Input: dimensioned drawing with shaded views. Units: mm. Origin: part minimum x, y, z. A direction names the side the tool comes from. Round coordinates to 2 decimals unless told otherwise and drop trailing zeros. Loops run counter-clockwise (first coordinate to the right, second up) from the corner with the lowest first, then second, coordinate; pieces in that order, holes last. Notation, with made-up numbers: M 34,33.5 L 41,33.5 A12 ccw 41,54.5 Z; hole C 88.25,20.25 d6. An arc over 180 degrees is marked long. Write each question's results on one line, items separated by ' | '. Start each with the question number.
1. Draft query along X for the marked faces 1, 2, 3 and 4. Return one class per face: released by +X, released by -X, zero draft, split by the parting line, or undercut.
2. Section A-A on z = 1. Output: boundary loops of the cut face in (x, y), and give its area (3 significant figures).
3. Section D-D on x = 9.75. Output: boundary loops of the cut face in (y, z), and give its area (3 significant figures).
4. Contact query for flat-ended pins moving along their axis: pin 1 Ø0.5 at (x, y) = (11.5, 8) entering from +Z; pin 2 Ø1.5 at (x, z) = (6.5, 6) entering from +Y; pin 3 Ø1.1 at (y, z) = (9.5, 2) entering from -X; pin 4 Ø3.5 at (x, y) = (5, 5) entering from -Z. Output: stop coordinate, or through.
5. Ray query, line 1 (X direction, y = 4.5, z = 4.75); line 2 (Z direction, x = 2.75, y = 8.5); line 3 (Y direction, x = 10, z = 3.25). Return the intervals inside material, ascending.
6. Section C-C on y = 7.75. Output: boundary loops of the cut face in (x, z).
7. Section B-B on x = 3.5. Output: boundary loops of the cut face in (y, z), and give its area (3 significant figures).
8. Set-up query: the marked faces 5, 6, 7, 8 and 9. Return all of +Z, -Z, +X, -X, +Y, -Y with unobstructed straight access to the full face (end or side cutting, diameter ignored); none if empty.
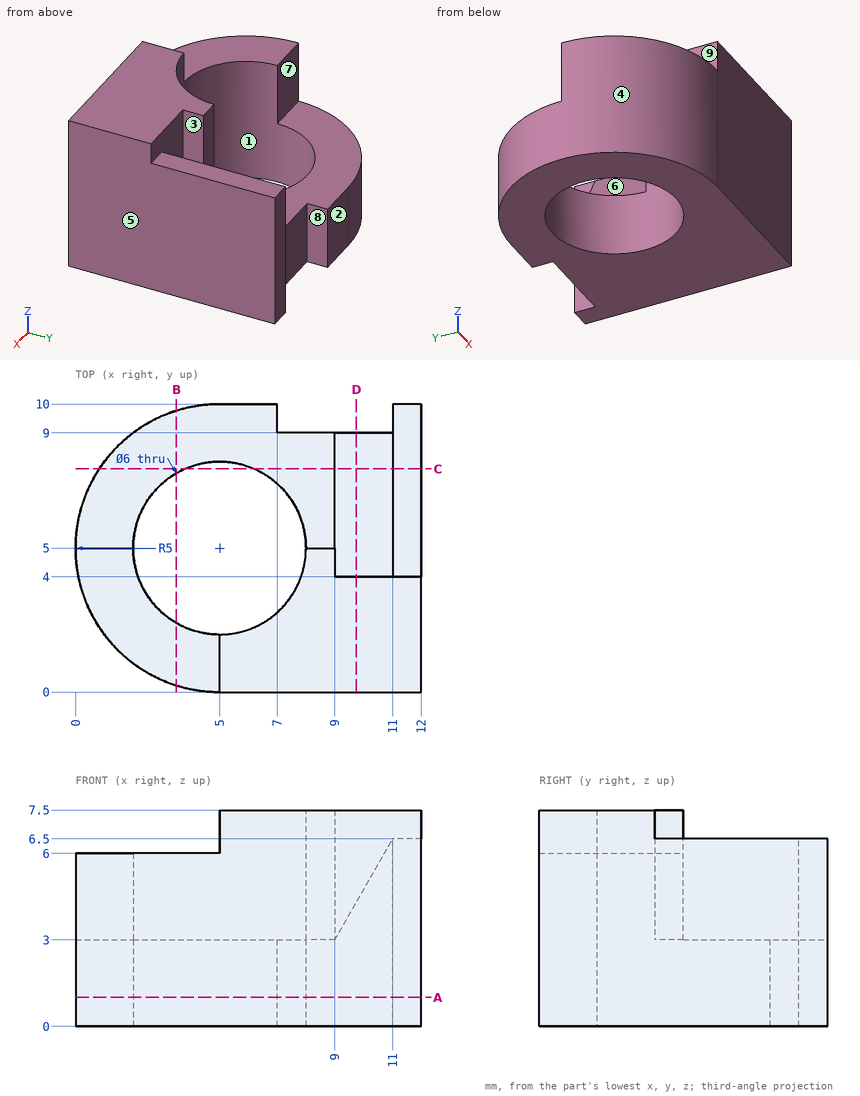
Taken from the geometry:
1) face 1: undercut | face 2: zero draft | face 3: undercut | face 4: released by -X
2) outline: M 5,0 L 12,0 L 12,10 L 11,10 L 11,9 L 7,9 L 7,10 L 5,10 A5 ccw Z; hole C 5,5 d6 | area: 77.0 mm^2
3) outline: M 0,0 L 9,0 L 9,4.31 L 4,4.31 L 4,7.5 L 0,7.5 Z | area: 51.6 mm^2
4) pin 1: z = 6.5 | pin 2: y = 3.02 | pin 3: x = 1.93 | pin 4: through
5) line 1: 0.03 to 2.04, 7.96 to 9, 10 to 12 | line 2: 0 to 3 | line 3: 0 to 9
6) outline: M 0.82,0 L 3.8,0 L 3.8,3 L 0.82,3 Z; M 6.2,0 L 12,0 L 12,6.5 L 11,6.5 L 9,3 L 6.2,3 Z
7) outline: M 0.23,0 L 2.4,0 L 2.4,6 L 0.23,6 Z; M 7.6,0 L 9.77,0 L 9.77,3 L 7.6,3 Z | area: 19.5 mm^2
8) face 5: +Z, -Z, +X, +Y, -Y | face 6: +Z, +Y | face 7: +Z, -X, +Y | face 8: +Z, -Z, +Y | face 9: +Z, -X, +Y, -Y
